Can you work these out from the model? Positions are in its coordinate system, mm. Face numbers are marked on the shaded views. A direction names the side the tool comes from. Coordinates: 2 decimals unless noted, no trailing zeros. Order: outer loops, then holes, each group sorted by start corner. A loop starts at its lowest first (then second) coordinate and runs counter-clockwise, first axis right, second up. Notation, with made-up numbers: (88.5, 21) -> (126.5, 21) arc R16 ccw to (126.5, 50) -> close; hole circle Ø3 at (66, -12.75). An arc over 180 degrees is marked (long way). Answer as CSV lines item,"result".
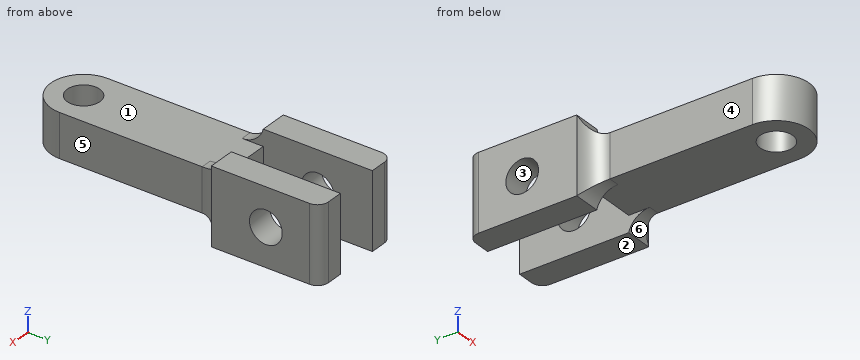
from build123d import *

# Parameters (mm, degrees)
SKETCH1_R           = 1.5
BOSS_EXTRUDE1_DEPTH = 4
SKETCH2_W           = 2.5
SKETCH2_H           = 7
BOSS_EXTRUDE2_DEPTH = 10
FILLET5_R           = 2
FILLET6_R           = 2
SKETCH3_R           = 1.5
CUT_EXTRUDE1_DEPTH  = 10
FILLET8_R           = 1


with BuildPart() as part:
    # Sketch1 → Boss-Extrude1 (new body)
    with BuildSketch(Plane.XY):
        with BuildLine():
            Line((-3, 0), (-3, 15))
            Line((-3, 15), (3, 15))
            Line((3, 15), (3, 0))
            ThreePointArc((3, 0), (0, -3), (-3, 0))
        make_face()
        Circle(SKETCH1_R, mode=Mode.SUBTRACT)
    extrude(amount=BOSS_EXTRUDE1_DEPTH)

    # Sketch2 → Boss-Extrude2 (add)
    with BuildSketch(Plane(origin=(0, 15, 0), x_dir=(1, 0, 0), z_dir=(0, 1, 0))):
        with Locations((3.25, -2)):
            Rectangle(SKETCH2_W, SKETCH2_H)
    boss_extrude2 = extrude(amount=BOSS_EXTRUDE2_DEPTH)

    # Mirror3: Boss-Extrude2 across plane
    add(boss_extrude2.mirror(Plane(origin=(0, 0, 0), x_dir=(0, 0, 1), z_dir=(1, 0, 0))))

    # Fillet5
    # the kernel refuses this fillet: 2 mm, written as the material it adds along each edge
    with BuildSketch(Plane(origin=(-3, 15, 4), x_dir=(0, 0, 1), z_dir=(1, 0, 0))) as fillet5_piece_1:
        with BuildLine():
            CenterArc((2, 1.936491673), FILLET5_R, 180, 75.522487814)
            Line((0, 1.936491673), (0, 0))
            Line((0, 0), (1.5, 0))
        make_face()
    extrude(amount=1)
    with BuildSketch(Plane(origin=(-3, 15, 0), x_dir=(0, 0, -1), z_dir=(1, 0, 0))) as fillet5_piece_2:
        with BuildLine():
            CenterArc((2, -1.936491673), FILLET5_R, 104.477512186, 75.522487814)
            Line((0, -1.936491673), (0, 0))
            Line((0, 0), (1.5, 0))
        make_face()
    extrude(amount=1)
    with BuildSketch(Plane(origin=(-3, 15, 0), x_dir=(0, -1, 0), z_dir=(0, 0, 1))) as fillet5_piece_3:
        with BuildLine():
            CenterArc((1.936491673, -2), FILLET5_R, 90, 75.522487814)
            Line((0, -1.5), (0, 0))
            Line((0, 0), (1.936491673, 0))
        make_face()
    extrude(amount=4)
    with BuildSketch(Plane(origin=(-3, 15, 0), x_dir=(0, -1, 0), z_dir=(0, 0, 1))) as fillet5_piece_4a_section:
        with BuildLine():
            CenterArc((1.936491673, -2), FILLET5_R, 90, 75.522487814)
            Line((0, -1.5), (0, 0))
            Line((0, 0), (1.936491673, 0))
        make_face()
    fillet5_piece_4a = extrude(amount=8.841229183, mode=Mode.PRIVATE)
    fillet5_piece_4a = split(fillet5_piece_4a, bisect_by=Plane(origin=(-3, 15, 4), z_dir=(0, 0, 1)), keep=Keep.TOP, mode=Mode.PRIVATE)
    fillet5_piece_4a = split(fillet5_piece_4a, bisect_by=Plane(origin=(-3, 15, 5.5), z_dir=(0, 0, -1)), keep=Keep.TOP, mode=Mode.PRIVATE)
    with BuildSketch(Plane(origin=(-7.841229183, 15, 4), x_dir=(0, 0, 1), z_dir=(1, 0, 0))) as fillet5_piece_4b_section:
        with BuildLine():
            CenterArc((2, 1.936491673), FILLET5_R, 180, 75.522487814)
            Line((0, 1.936491673), (0, 0))
            Line((0, 0), (1.5, 0))
        make_face()
    fillet5_piece_4b = extrude(amount=5.841229183, mode=Mode.PRIVATE)
    fillet5_piece_4b = split(fillet5_piece_4b, bisect_by=Plane(origin=(-3, 15, 4), z_dir=(-1, 0, 0)), keep=Keep.TOP, mode=Mode.PRIVATE)
    fillet5_piece_4b = split(fillet5_piece_4b, bisect_by=Plane(origin=(-4.5, 15, 4), z_dir=(1, 0, 0)), keep=Keep.TOP, mode=Mode.PRIVATE)
    fillet5_piece_4 = fillet5_piece_4a & fillet5_piece_4b
    add(fillet5_piece_4)
    with BuildSketch(Plane(origin=(-3, 15, -4.841229183), x_dir=(0, -1, 0), z_dir=(0, 0, 1))) as fillet5_piece_5a_section:
        with BuildLine():
            CenterArc((1.936491673, -2), FILLET5_R, 90, 75.522487814)
            Line((0, -1.5), (0, 0))
            Line((0, 0), (1.936491673, 0))
        make_face()
    fillet5_piece_5a = extrude(amount=8.841229183, mode=Mode.PRIVATE)
    fillet5_piece_5a = split(fillet5_piece_5a, bisect_by=Plane(origin=(-3, 15, 0), z_dir=(0, 0, -1)), keep=Keep.TOP, mode=Mode.PRIVATE)
    fillet5_piece_5a = split(fillet5_piece_5a, bisect_by=Plane(origin=(-3, 15, -1.5), z_dir=(0, 0, 1)), keep=Keep.TOP, mode=Mode.PRIVATE)
    with BuildSketch(Plane(origin=(-7.841229183, 15, 0), x_dir=(0, 0, -1), z_dir=(1, 0, 0))) as fillet5_piece_5b_section:
        with BuildLine():
            CenterArc((2, -1.936491673), FILLET5_R, 104.477512186, 75.522487814)
            Line((0, -1.936491673), (0, 0))
            Line((0, 0), (1.5, 0))
        make_face()
    fillet5_piece_5b = extrude(amount=5.841229183, mode=Mode.PRIVATE)
    fillet5_piece_5b = split(fillet5_piece_5b, bisect_by=Plane(origin=(-3, 15, 0), z_dir=(-1, 0, 0)), keep=Keep.TOP, mode=Mode.PRIVATE)
    fillet5_piece_5b = split(fillet5_piece_5b, bisect_by=Plane(origin=(-4.5, 15, 0), z_dir=(1, 0, 0)), keep=Keep.TOP, mode=Mode.PRIVATE)
    fillet5_piece_5 = fillet5_piece_5a & fillet5_piece_5b
    add(fillet5_piece_5)

    # Fillet6
    # the kernel refuses this fillet: 2 mm, written as the material it adds along each edge
    with BuildSketch(Plane(origin=(2, 15, 4), x_dir=(0, -1, 0), z_dir=(1, 0, 0))) as fillet6_piece_1:
        with BuildLine():
            CenterArc((1.936491673, -2), FILLET6_R, 90, 75.522487814)
            Line((0, -1.5), (0, 0))
            Line((0, 0), (1.936491673, 0))
        make_face()
    extrude(amount=1)
    with BuildSketch(Plane(origin=(2, 15, 0), x_dir=(0, 0, -1), z_dir=(1, 0, 0))) as fillet6_piece_2:
        with BuildLine():
            CenterArc((2, -1.936491673), FILLET6_R, 104.477512186, 75.522487814)
            Line((0, -1.936491673), (0, 0))
            Line((0, 0), (1.5, 0))
        make_face()
    extrude(amount=1)
    with BuildSketch(Plane(origin=(3, 15, 0), x_dir=(1, 0, 0), z_dir=(0, 0, 1))) as fillet6_piece_3:
        with BuildLine():
            CenterArc((2, -1.936491673), FILLET6_R, 104.477512186, 75.522487814)
            Line((0, -1.936491673), (0, 0))
            Line((0, 0), (1.5, 0))
        make_face()
    extrude(amount=4)
    with BuildSketch(Plane(origin=(2, 15, 4), x_dir=(0, -1, 0), z_dir=(1, 0, 0))) as fillet6_piece_4a_section:
        with BuildLine():
            CenterArc((1.936491673, -2), FILLET6_R, 90, 75.522487814)
            Line((0, -1.5), (0, 0))
            Line((0, 0), (1.936491673, 0))
        make_face()
    fillet6_piece_4a = extrude(amount=5.841229183, mode=Mode.PRIVATE)
    fillet6_piece_4a = split(fillet6_piece_4a, bisect_by=Plane(origin=(4.5, 15, 4), z_dir=(-1, 0, 0)), keep=Keep.TOP, mode=Mode.PRIVATE)
    fillet6_piece_4a = split(fillet6_piece_4a, bisect_by=Plane(origin=(3, 15, 4), z_dir=(1, 0, 0)), keep=Keep.TOP, mode=Mode.PRIVATE)
    with BuildSketch(Plane(origin=(3, 15, 0), x_dir=(1, 0, 0), z_dir=(0, 0, 1))) as fillet6_piece_4b_section:
        with BuildLine():
            CenterArc((2, -1.936491673), FILLET6_R, 104.477512186, 75.522487814)
            Line((0, -1.936491673), (0, 0))
            Line((0, 0), (1.5, 0))
        make_face()
    fillet6_piece_4b = extrude(amount=8.841229183, mode=Mode.PRIVATE)
    fillet6_piece_4b = split(fillet6_piece_4b, bisect_by=Plane(origin=(3, 15, 4), z_dir=(0, 0, 1)), keep=Keep.TOP, mode=Mode.PRIVATE)
    fillet6_piece_4b = split(fillet6_piece_4b, bisect_by=Plane(origin=(3, 15, 5.5), z_dir=(0, 0, -1)), keep=Keep.TOP, mode=Mode.PRIVATE)
    fillet6_piece_4 = fillet6_piece_4a & fillet6_piece_4b
    add(fillet6_piece_4)
    with BuildSketch(Plane(origin=(2, 15, 0), x_dir=(0, 0, -1), z_dir=(1, 0, 0))) as fillet6_piece_5a_section:
        with BuildLine():
            CenterArc((2, -1.936491673), FILLET6_R, 104.477512186, 75.522487814)
            Line((0, -1.936491673), (0, 0))
            Line((0, 0), (1.5, 0))
        make_face()
    fillet6_piece_5a = extrude(amount=5.841229183, mode=Mode.PRIVATE)
    fillet6_piece_5a = split(fillet6_piece_5a, bisect_by=Plane(origin=(4.5, 15, 0), z_dir=(-1, 0, 0)), keep=Keep.TOP, mode=Mode.PRIVATE)
    fillet6_piece_5a = split(fillet6_piece_5a, bisect_by=Plane(origin=(3, 15, 0), z_dir=(1, 0, 0)), keep=Keep.TOP, mode=Mode.PRIVATE)
    with BuildSketch(Plane(origin=(3, 15, -4.841229183), x_dir=(1, 0, 0), z_dir=(0, 0, 1))) as fillet6_piece_5b_section:
        with BuildLine():
            CenterArc((2, -1.936491673), FILLET6_R, 104.477512186, 75.522487814)
            Line((0, -1.936491673), (0, 0))
            Line((0, 0), (1.5, 0))
        make_face()
    fillet6_piece_5b = extrude(amount=8.841229183, mode=Mode.PRIVATE)
    fillet6_piece_5b = split(fillet6_piece_5b, bisect_by=Plane(origin=(3, 15, -1.5), z_dir=(0, 0, 1)), keep=Keep.TOP, mode=Mode.PRIVATE)
    fillet6_piece_5b = split(fillet6_piece_5b, bisect_by=Plane(origin=(3, 15, 0), z_dir=(0, 0, -1)), keep=Keep.TOP, mode=Mode.PRIVATE)
    fillet6_piece_5 = fillet6_piece_5a & fillet6_piece_5b
    add(fillet6_piece_5)

    # Sketch3 → Cut-Extrude1 (cut)
    with BuildSketch(Plane.ZY.offset(4.5)):
        with Locations((2, 20)):
            Circle(SKETCH3_R)
    extrude(amount=-CUT_EXTRUDE1_DEPTH, mode=Mode.SUBTRACT)

    # Fillet8
    fillet8_edges = [part.edges().sort_by_distance(p)[0] for p in [
        (4.5, 25, 2),
        (-4.5, 25, 2),
    ]]
    fillet(fillet8_edges, radius=FILLET8_R)


solid = part.part
Q1. Imagine slicing it at D-D (z = 2). List the corners of the cut face in (x, y) for me, and give its area (3 significant figures).
Solution:
outline,"(-4.5, 15) arc R2 cw to (-3, 13.06) -> (-3, 0) arc R3 ccw to (3, 0) -> (3, 13.06) arc R2 cw to (4.5, 15) -> (4.5, 18.5) -> (2, 18.5) -> (2, 15) -> (-2, 15) -> (-2, 18.5) -> (-4.5, 18.5) -> close; (-4.5, 21.5) -> (-2, 21.5) -> (-2, 25) -> (-3.5, 25) arc R1 ccw to (-4.5, 24) -> close; (2, 21.5) -> (4.5, 21.5) -> (4.5, 24) arc R1 ccw to (3.5, 25) -> (2, 25) -> close; hole circle Ø3 at (0, 0)"
area,"133 mm2"
Q2. We'd pull the mould along Z, two halves only. Please class the marked faces 1, 2 and 3: pulls with the +Z half, pulls with the -Z half, needs draft (parallel to the pull), parting line crosses it, or undercut.
Solution:
face 1,"pulls with the +Z half"
face 2,"pulls with the -Z half"
face 3,"undercut"
Q3. Imagine slicing it at B-B (z = 0.75). List the corners of the cut face in (x, y) for me, and give its area (3 significant figures).
Solution:
outline,"(-4.5, 15) arc R2 cw to (-3, 13.06) -> (-3, 0) arc R3 ccw to (3, 0) -> (3, 13.06) arc R2 cw to (4.5, 15) -> (4.5, 19.17) -> (2, 19.17) -> (2, 15) -> (-2, 15) -> (-2, 19.17) -> (-4.5, 19.17) -> close; (-4.5, 20.83) -> (-2, 20.83) -> (-2, 25) -> (-3.5, 25) arc R1 ccw to (-4.5, 24) -> close; (2, 20.83) -> (4.5, 20.83) -> (4.5, 24) arc R1 ccw to (3.5, 25) -> (2, 25) -> close; hole circle Ø3 at (0, 0)"
area,"140 mm2"
Q4. Imagine slicing it at A-A (y = 20). List the corners of the cut face in (x, z) for me, and give its area (3 significant figures).
Solution:
outline,"(-4.5, -1.5) -> (-2, -1.5) -> (-2, 0.5) -> (-4.5, 0.5) -> close; (-4.5, 3.5) -> (-2, 3.5) -> (-2, 5.5) -> (-4.5, 5.5) -> close; (2, -1.5) -> (4.5, -1.5) -> (4.5, 0.5) -> (2, 0.5) -> close; (2, 3.5) -> (4.5, 3.5) -> (4.5, 5.5) -> (2, 5.5) -> close"
area,"20.0 mm2"
Q5. For P1, Ø1.8, axis at x = -0.5, y = 6, coming from the -Z side; P2, Ø1, axis at x = 0, z = 1.5, coming from the +Y side; P3, Ø2, axis at x = -3.5, z = 2.5, coming from the -Y side, each with a flat end and sliding along its axis, tell me the tip position at first contact or that it passes through.
Solution:
P1,"z = 0"
P2,"y = 15"
P3,"y = -1.66"
Q6. Which directions (+Z, -Z, +X, -X, +Y, -Y) give clear straight access to the entire face, cutting with the end or side of a thin tool? Please do the marked faces 4, 5 and 6.
Solution:
face 4,"+Z, -Z, -X, -Y"
face 5,"+Z, -Z, +X, -Y"
face 6,"-Z, +X, -X, -Y"
Q7. If I drill on line 1 (X direction, y = 17, z = 3.5); line 2 (Y direction, x = 0, z = 1.25); line 3 (X direction, y = 11.25, z = 2.25), over which ranges is the centre line in solid material (lowest first)?
Solution:
line 1,"-4.5 to -2, 2 to 4.5"
line 2,"-3 to -1.5, 1.5 to 15"
line 3,"-3 to 3"
Q8. Imagine slicing it at C-C (x = 0). List the corners of the cut face in (y, z) for me.
Solution:
outline,"(-3, 0) -> (-1.5, 0) -> (-1.5, 4) -> (-3, 4) -> close; (1.5, 0) -> (15, 0) -> (15, 4) -> (1.5, 4) -> close"
